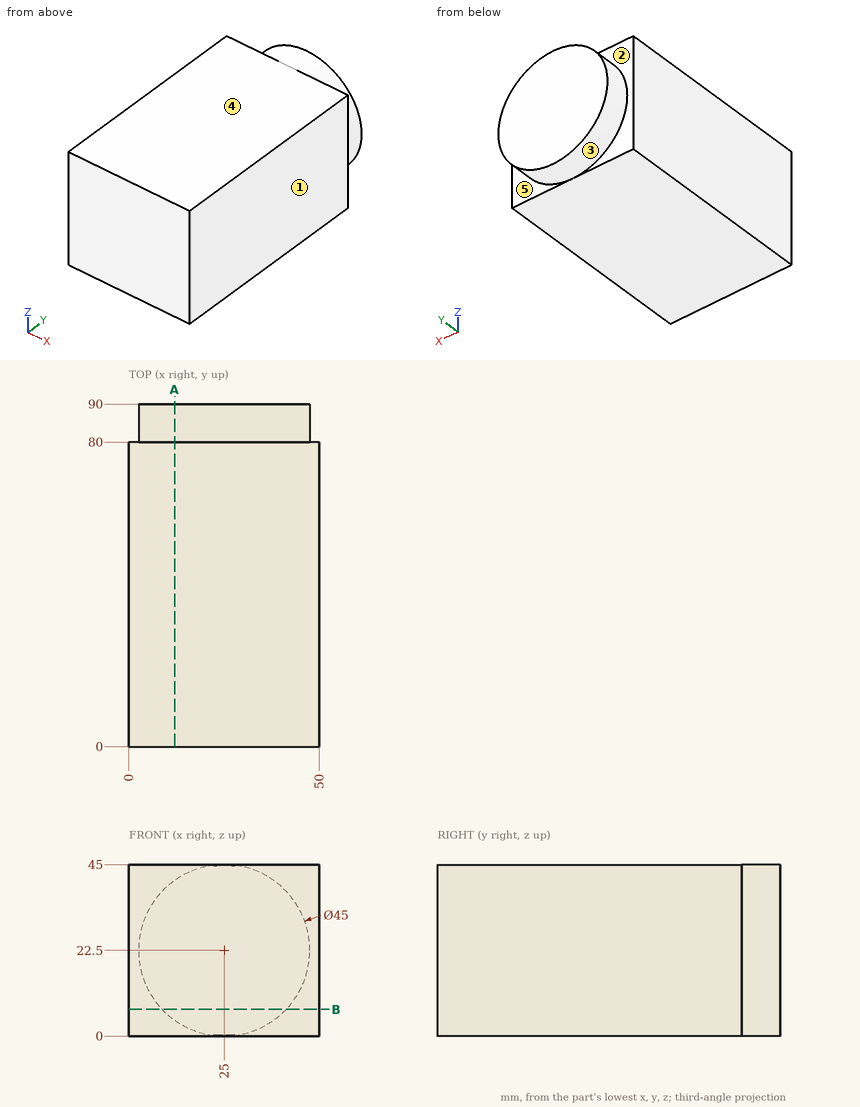
Answer from the drawing. Dimensions are ordinates in mm from the lowest x, y and z of the part. A direction names the side the tool comes from. Give positions to 0.01 mm unless a question says otherwise; leave off trailing zeros. Loops run counter-clockwise (first coordinate to the right, second up) from the corner with the lowest first, then second, coordinate; pieces in that order, holes last. Notation, with made-up numbers: (81, 83.5) - (96, 83.5) arc R12 cw to (96, 102.5) - close; hole circle Ø8 at (-26.75, 54.25). An arc over 180 degrees is marked (long way). Answer as CSV lines item,"result". Start each with the question number.
Item 1: A cutting plane is placed at B-B on z = 7. Determine the outline of the cut face in (x, y).
Item 2: For the marked faces 1, 2, 3, 4 and 5, determine the directions among +Z, -Z, +X, -X, +Y, -Y from which every point of the face is accessible in a straight line to the end or side of a thin tool.
Item 3: Find the intervals of material crossed by line 1 (Y direction, x = 4.5, z = 35.5); line 2 (X direction, y = 85.5, z = 14.5); line 3 (Z direction, x = 26, y = 83), in increasing order. Write a range as from..to.
Item 4: A cutting plane is placed at A-A on x = 12. Determine the outline of the cut face in (y, z).
Found:
1,outline,"(0, 0) - (50, 0) - (50, 80) - (41.31, 80) - (41.31, 90) - (8.69, 90) - (8.69, 80) - (0, 80) - close"
2,face 1,"+Z, -Z, +X, +Y, -Y"
2,face 2,"-X, +Y"
2,face 3,"+Y"
2,face 4,"+Z, +X, -X, +Y, -Y"
2,face 5,"+X, +Y"
3,line 1,"y = 0..80"
3,line 2,"x = 3.97..46.03"
3,line 3,"z = 0.02..44.98"
4,outline,"(0, 0) - (80, 0) - (80, 4.14) - (90, 4.14) - (90, 40.86) - (80, 40.86) - (80, 45) - (0, 45) - close"
